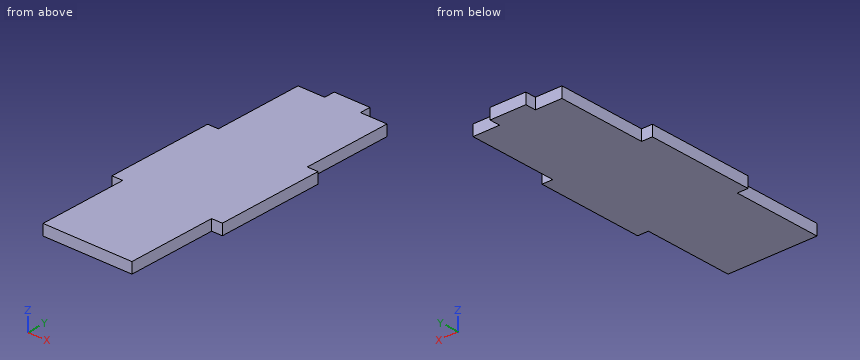
from build123d import *

# Parameters (mm, degrees)
EXTRUDE_1_DEPTH = 3


with BuildPart() as part:
    # 草图1 → 凸台-拉伸1 (new body)
    with BuildSketch(Plane.XY):
        Polygon((0, -25), (0, -40), (12.435, -40), (12.435, 0), (7.435, 0), (0, 0), align=None)
        Polygon((12.435, 0), (12.435, -40), (24.87, -40), (24.87, -25), (24.87, 0), (17.435, 0), align=None)
        Polygon((24.87, -40), (12.435, -40), (12.435, -80), (24.87, -80), (24.87, -55), align=None)
        Polygon((12.435, -40), (0, -40), (0, -55), (0, -80), (12.435, -80), align=None)
        Polygon((0, -55), (0, -40), (0, -25), (-3, -25), (-3, -55), align=None)
        Polygon((7.435, 0), (12.435, 0), (17.435, 0), (17.435, 3), (7.435, 3), align=None)
        Polygon((24.87, -25), (24.87, -40), (24.87, -55), (27.87, -55), (27.87, -25), align=None)
    extrude(amount=EXTRUDE_1_DEPTH)


solid = part.part
Source: CAD feature listing. Evaluate the final solid. Frame: model axes, mm. Give positions to 0.01 mm unless a question says otherwise; leave off trailing zeros. Order: outer loops, then holes, each group sorted by start corner. A loop starts at its lowest first (then second) coordinate and runs counter-clockwise, first axis right, second up. Notation, with made-up numbers: (68, 8) -> (127, 8) arc R30 cw to (127, 44) -> close; hole circle Ø9 at (69, -0.75). An arc over 180 degrees is marked (long way). Write item = value, one per line.
Item 1: Section query A-A (z = 1.8). Output: boundary loops of the cut face in (x, y) (3 decimals).
Check result:
outline = (-3, -55) -> (0, -55) -> (0, -80) -> (24.87, -80) -> (24.87, -55) -> (27.87, -55) -> (27.87, -25) -> (24.87, -25) -> (24.87, 0) -> (17.435, 0) -> (17.435, 3) -> (7.435, 3) -> (7.435, 0) -> (0, 0) -> (0, -25) -> (-3, -25) -> close
Item 2: Section query B-B (x = 19). Output: boundary loops of the cut face in (y, z), then the cut area to 3 significant figures.
Check result:
outline = (-80, 0) -> (0, 0) -> (0, 3) -> (-80, 3) -> close
area = 240 mm²
Item 3: Ray query, probe 1 along Y at (x, z) = (7, 1.4); probe 2 along X at (y, z) = (-2, 2.85). Return the intervals inside material, ascending.
Check result:
probe_1 = -80 to 0
probe_2 = 0 to 24.87
Item 4: Contact query for flat-ended pins moving along their axis: pin 1 (1.5 mm diameter, centred on y = -10.5, z = 1.5, fed in from +X); pin 2 (1.5 mm diameter, centred on y = 1, z = 1, fed in from -X) (3 decimals); pin 3 (0.9 mm diameter, centred on x = 26.5, z = 2, fed in from -Y); pin 4 (12 mm diameter, centred on x = 18.5, y = -19, fed in from -Z). Output: stop coordinate, or through.
Check result:
pin_1 = 24.87
pin_2 = 7.435
pin_3 = -55
pin_4 = 0
Item 5: Section query C-C (y = -22). Output: boundary loops of the cut face in (x, z), then the cut area to 3 significant figures.
Check result:
outline = (0, 0) -> (24.87, 0) -> (24.87, 3) -> (0, 3) -> close
area = 74.6 mm²
